CAD build for the part. Positions are in the model's coordinates, mm. Face numbers are marked on the shaded views. A direction names the side the tool comes from. Coordinates: 2 decimals unless noted, no trailing zeros. Loops run counter-clockwise (first coordinate to the right, second up) from the corner with the lowest first, then second, coordinate; pieces in that order, holes last. Notation, with made-up numbers: (87.5, 37) - (121.5, 37) arc R33 cw to (121.5, 67) - close; hole circle Ø2 at (-10, 25.25). An arc over 180 degrees is marked (long way). Put each result on its own line as item: value.
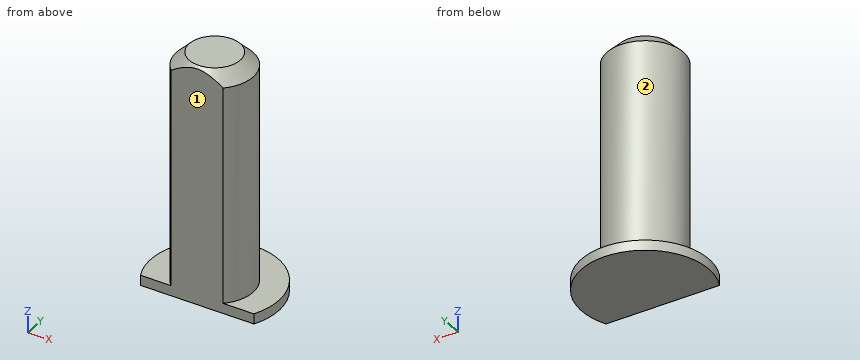
Autodesk Inventor part; units mm, degrees
ref_plane "YZ Plane" through (0, 0, 0) normal (1, 0, 0) x (0, 1, 0)
ref_plane "XZ Plane" through (0, 0, 0) normal (0, 1, 0) x (-1, 0, 0)
ref_plane "XY Plane" through (0, 0, 0) normal (0, 0, 1) x (1, 0, 0)
sketch "Sketch1" plane through (0, 0, 0) normal (0, 0, 1) x (1, 0, 0)
  circle A0 centre (0, 0) radius 1.5
  dimension "d0" = 3
extrude "Extrusion1" add sketch "Sketch1" along normal blind 9
sketch "Sketch2" plane through (0, 0, 0) normal (0, 0, -1) x (-1, 0, 0)
  circle A0 centre (0, 0) radius 1.5 construction
  circle A1 centre (0, 0) radius 2.5
  dimension "d3" = 5
extrude "Extrusion2" add sketch "Sketch2" along normal blind 0.4
chamfer "Chamfer1" distance 0.5 angle 45 1 edges at (-1.5, 0, 9)
sketch "Sketch3" plane through (0, 0, -0.4) normal (0, 0, -1) x (-1, 0, 0)
  circle A0 centre (0, 0) radius 1.5 construction
  circle A1 centre (0, 0) radius 2.5
  line L0 (-2.25, -1.0897) -> (2.25, -1.0897)
  dimension "d9" = 4.5
extrude "Extrusion3" cut sketch "Sketch3" against normal through all contours L0 A1 picked at (-0.1034, -1.5534)
properties part number "Spring_pin"
Q1. Slice it at D-D, the plane x = -1.8. Give the cut face in (y, z), then the cut area to 3 significant figures.
Determined:
outline: (-1.09, -0.4) - (1.73, -0.4) - (1.73, 0) - (-1.09, 0) - close
area: 1.13 mm2
Q2. Wall check: L1, parallel to Z at x = 1.9, y = 0.3; L2, parallel to Y at x = 0.05, z = 7; L3, parallel to Z at x = -1.2, y = -0.7. Give the ranges that are in metal, low to high. Write a range as from..to.
Determined:
L1: -0.4..0
L2: -1.09..1.5
L3: -0.4..8.61
Q3. Slice it at B-B, the plane y = 0. Give the cut face in (x, z).
Determined:
outline: (-2.5, -0.4) - (2.5, -0.4) - (2.5, 0) - (1.5, 0) - (1.5, 8.5) - (1, 9) - (-1, 9) - (-1.5, 8.5) - (-1.5, 0) - (-2.5, 0) - close
Q4. Slice it at A-A, the plane x = 0. Give the cut face in (y, z).
Determined:
outline: (-1.09, -0.4) - (2.5, -0.4) - (2.5, 0) - (1.5, 0) - (1.5, 8.5) - (1, 9) - (-1, 9) - (-1.09, 8.91) - close
Q5. Tool access for the marked faces 1 and 2: list every direction of +Z, -Z, +X, -X, +Y, -Y with a clear straight run to the whole face (end or side of a thin tool).
Determined:
face 1: +Z, -Z, +X, -X, -Y
face 2: +Z
Q6. Pin check, flat tips, straight feed: pin 1 Ø1.5 at (x, z) = (-2, 6) entering from +Y; pin 2 Ø1.5 at (y, z) = (1.5, 4) entering from -X; pin 3 Ø1.5 at (y, z) = (2, 6) entering from -X. Stop position of each tip, or through.
Determined:
pin 1: y = 0.83
pin 2: x = -1.3
pin 3: x = -0.83
Q7. Slice it at C-C, the plane z = 6.25. Give the cut face in (x, y).
Determined:
outline: (-1.03, -1.09) - (1.03, -1.09) arc R1.5 ccw (long way) to start
